For this review, take the finished solid that the model builds, in its own axes (mm). A direction names the side the tool comes from. Coordinates: 2 decimals unless noted, no trailing zeros. Order: outer loops, then holes, each group sorted by start corner. A loop starts at its lowest first (then second) coordinate and runs counter-clockwise, first axis right, second up. Notation, with made-up numbers: (-36.75, 34) -> (-16.75, 34) arc R28 cw to (-16.75, 72) -> close; hole circle Ø2 at (65.25, -10). An arc over 180 degrees is marked (long way). Write item = value, one per line. Start each with the question number.
1) Consider section A-A on x = -17.5. Give the boundary of the cut face in (y, z).
2) Consider section B-B on y = 22. Give the boundary of the cut face in (x, z).
3) Consider section C-C on x = 2. Give the boundary of the cut face in (y, z).
4) Draft analysis for pull direction X (two halves, no side actions). For faces 3 (the face through (57, 35.501, 15)), 4 (the face through (66.93, 42.4, -0.99)), 5 (the face through (-3.825, 36.621, 14.79)), state which applies: +X half, -X half, draft (parallel to the pull), parting line (faces both ways), or undercut.
5) Machinability: for faces 1 (the face through (66.9, -2.43, -0.99)), 2 (the face through (2, 40, 0)), which of the approach directions +Z, -Z, +X, -X, +Y, -Y give a long, thin tool a straight path to every point of the face, cutting with its end or side? Answer none if there is none.
6) Wall thickness on probe 1 along Y at (x, z) = (2, 2.6); probe 2 along X at (y, z) = (5.5, 19.5); probe 3 along Y at (x, z) = (43, 24): over which ranges is each line inside the solid? List them lowest first. Write a range as [from, to].
7) Insertion check: pin 1 Ø12 at (y, z) = (34.5, 8) entering from +X; pin 2 Ø9 at (y, z) = (25, 21.5) entering from +X; pin 3 Ø3 at (x, y) = (50.5, 39.5) entering from +Z; pin 4 Ø4 at (x, y) = (62.5, 22) entering from -Z. Each pin has a flat end and moves straight along its axis. Give the tip position at first contact, or say it passes through.
8) Consider section D-D on y = 33. Give the boundary of the cut face in (x, z).
from build123d import *

# Parameters (mm, degrees)
SKETCH_2_R          = 3.25
EXTRUDE_1_DEPTH     = 2
SKETCH_2_3_R        = 2
EXTRUDE_2_DEPTH     = 30
SKETCH_2_4_R        = 1.6
EXTRUDE_3_DEPTH     = 4
CUT_EXTRUDE_1_REACH = 80
SKETCH_3_R          = 2.5
SKETCH_3_R_2        = 2
CUT_EXTRUDE_2_REACH = 3.5


with BuildPart() as part:
    # Sketch 2 → Extrude 1 (new body)
    with BuildSketch(Plane.XY):
        with BuildLine():
            ThreePointArc((-20.5, 43.00095784), (-21.914213562, 42.415171403), (-22.5, 41.00095784))
            Line((-22.5, 41.00095784), (-22.5, -1))
            ThreePointArc((-22.5, -1), (-21.914213562, -2.414213562), (-20.5, -3))
            Line((-20.5, -3), (65.5, -3))
            ThreePointArc((65.5, -3), (66.914213562, -2.414213562), (67.5, -1))
            Line((67.5, -1), (67.5, 41.00095784))
            ThreePointArc((67.5, 41.00095784), (66.914213562, 42.415171403), (65.5, 43.00095784))
            Line((65.5, 43.00095784), (-20.5, 43.00095784))
        make_face()
        with Locations((-17.5, 22)):
            Circle(SKETCH_2_R, mode=Mode.SUBTRACT)
        with Locations((62.5, 22)):
            Circle(SKETCH_2_R, mode=Mode.SUBTRACT)
    extrude(amount=-EXTRUDE_1_DEPTH)

    # Sketch 2_3 → Extrude 2 (add)
    with BuildSketch(Plane.XY):
        with BuildLine():
            ThreePointArc((-10.601500464, -1), (-10.015714027, -2.414213562), (-8.601500464, -3))
            Line((-8.601500464, -3), (57.5, -3))
            ThreePointArc((57.5, -3), (61.5, 1), (57.5, 5))
            Line((57.5, 5), (55.5, 5))
            Line((55.5, 5), (55.5, 35.50095784))
            Line((55.5, 35.50095784), (58.590729836, 35.50095784))
            ThreePointArc((58.590729836, 35.50095784), (62.463713182, 38.50095784), (60.527221509, 43.00095784))
            Line((60.527221509, 43.00095784), (-8.601500464, 43.00095784))
            ThreePointArc((-8.601500464, 43.00095784), (-10.015714027, 42.415171403), (-10.601500464, 41.00095784))
            Line((-10.601500464, 41.00095784), (-10.601500464, -1))
        make_face()
        with Locations((-6.601500464, 1)):
            Circle(SKETCH_2_3_R, mode=Mode.SUBTRACT)
        with BuildLine():
            ThreePointArc((-3.137398849, -1), (-3.77307334, 3.828427125), (-8.601500464, 4.464101615))
            Line((-8.601500464, 4.464101615), (-8.601500464, 36.036856225))
            ThreePointArc((-8.601500464, 36.036856225), (-3.77307334, 36.672530716), (-3.137398849, 41.50095784))
            Line((-3.137398849, 41.50095784), (53.5, 41.50095784))
            Line((53.5, 41.50095784), (53.5, -1))
            Line((53.5, -1), (-3.137398849, -1))
        make_face(mode=Mode.SUBTRACT)
        with Locations((-6.601500464, 39.50095784)):
            Circle(SKETCH_2_3_R, mode=Mode.SUBTRACT)
        with Locations((57.5, 1)):
            Circle(SKETCH_2_3_R, mode=Mode.SUBTRACT)
        with Locations((58.590729836, 39.50095784)):
            Circle(SKETCH_2_3_R, mode=Mode.SUBTRACT)
    extrude(amount=EXTRUDE_2_DEPTH)

    # Sketch 2_4 → Extrude 3 (add)
    with BuildSketch(Plane.XY):
        with BuildLine():
            Line((4.872781496, 41.50095784), (-0.872781496, 41.50095784))
            ThreePointArc((-0.872781496, 41.50095784), (2, 35.99904216), (4.872781496, 41.50095784))
        make_face()
        with Locations((2, 39.5)):
            Circle(SKETCH_2_4_R, mode=Mode.SUBTRACT)
        with BuildLine():
            ThreePointArc((4.645751311, -1), (2, 6), (-0.645751311, -1))
            Line((-0.645751311, -1), (4.645751311, -1))
        make_face()
        with Locations((2, 2)):
            Circle(SKETCH_2_4_R, mode=Mode.SUBTRACT)
        with BuildLine():
            ThreePointArc((47.627218504, 41.50095784), (48.596140902, 36.56196897), (53.5, 37.695365466))
            Line((53.5, 37.695365466), (53.5, 41.50095784))
            Line((53.5, 41.50095784), (47.627218504, 41.50095784))
        make_face()
        with Locations((50.5, 39.5)):
            Circle(SKETCH_2_4_R, mode=Mode.SUBTRACT)
        with BuildLine():
            ThreePointArc((53.5, 4.645751311), (47.671572875, 4.828427125), (47.854248689, -1))
            Line((47.854248689, -1), (53.5, -1))
            Line((53.5, -1), (53.5, 4.645751311))
        make_face()
        with Locations((50.5, 2)):
            Circle(SKETCH_2_4_R, mode=Mode.SUBTRACT)
    extrude(amount=EXTRUDE_3_DEPTH)

    # Sketch 3 → Cut-Extrude 1 (cut, up to next)
    with BuildSketch(Plane(origin=(55.5, 0, 0), x_dir=(0, 0, -1), z_dir=(1, 0, 0)), mode=Mode.PRIVATE) as cut_extrude_1_sk1:
        with Locations((-30, 12.50095784)):
            Circle(SKETCH_3_R)
    cut_extrude_1_tool1 = extrude(cut_extrude_1_sk1.sketch, amount=-CUT_EXTRUDE_1_REACH, mode=Mode.PRIVATE) & part.part
    add(cut_extrude_1_tool1.solids().sort_by_distance((55.5, 12.500958, 30))[0], mode=Mode.SUBTRACT)
    # Sketch 3 → Cut-Extrude 1 (cut, up to next)
    with BuildSketch(Plane(origin=(55.5, 0, 0), x_dir=(0, 0, -1), z_dir=(1, 0, 0)), mode=Mode.PRIVATE) as cut_extrude_1_sk2:
        with Locations((-30, 28.50095784)):
            Circle(SKETCH_3_R_2)
    cut_extrude_1_tool2 = extrude(cut_extrude_1_sk2.sketch, amount=-CUT_EXTRUDE_1_REACH, mode=Mode.PRIVATE) & part.part
    add(cut_extrude_1_tool2.solids().sort_by_distance((55.5, 28.500958, 30))[0], mode=Mode.SUBTRACT)

    # Sketch 5 → Cut-Extrude 2 (cut, up to next)
    with BuildSketch(Plane.XZ.offset(-41.50095784), mode=Mode.PRIVATE) as cut_extrude_2_sk1:
        with BuildLine():
            Line((39.27567, 8.8), (47.49867, 8.8))
            Line((47.49867, 8.8), (47.49867, 6.3))
            ThreePointArc((47.49867, 6.3), (47.205776781, 5.592893219), (46.49867, 5.3))
            Line((46.49867, 5.3), (40.27567, 5.3))
            ThreePointArc((40.27567, 5.3), (39.568563219, 5.592893219), (39.27567, 6.3))
            Line((39.27567, 6.3), (39.27567, 8.8))
        make_face()
    cut_extrude_2_tool1 = extrude(cut_extrude_2_sk1.sketch, amount=-CUT_EXTRUDE_2_REACH, mode=Mode.PRIVATE) & part.part
    add(cut_extrude_2_tool1.solids().sort_by_distance((43.38717, 41.500958, 7.073111))[0], mode=Mode.SUBTRACT)


solid = part.part
Answer sheet:
q1.outline = (-3, -2) -> (18.75, -2) -> (18.75, 0) -> (-3, 0) -> close; (25.25, -2) -> (43, -2) -> (43, 0) -> (25.25, 0) -> close
q2.outline = (-22.5, -2) -> (-20.75, -2) -> (-20.75, 0) -> (-22.5, 0) -> close; (-14.25, -2) -> (59.25, -2) -> (59.25, 0) -> (55.5, 0) -> (55.5, 30) -> (53.5, 30) -> (53.5, 0) -> (-8.6, 0) -> (-8.6, 30) -> (-10.6, 30) -> (-10.6, 0) -> (-14.25, 0) -> close; (65.75, -2) -> (67.5, -2) -> (67.5, 0) -> (65.75, 0) -> close
q3.outline = (-3, -2) -> (43, -2) -> (43, 30) -> (41.5, 30) -> (41.5, 4) -> (41.1, 4) -> (41.1, 0) -> (37.9, 0) -> (37.9, 4) -> (36, 4) -> (36, 0) -> (6, 0) -> (6, 4) -> (3.6, 4) -> (3.6, 0) -> (0.4, 0) -> (0.4, 4) -> (-1, 4) -> (-1, 30) -> (-3, 30) -> close
q4.face_3 = draft
q4.face_4 = +X half
q4.face_5 = undercut
q5.face_1 = +Z, -Z, +X, -Y
q5.face_2 = +Z
q6.probe_1 = [-3, 0.4], [3.6, 6], [36, 37.9], [41.1, 43]
q6.probe_2 = [-10.6, -8.6], [53.5, 55.5]
q6.probe_3 = [-3, -1], [41.5, 43]
q7.pin_1 = 62.59
q7.pin_2 = 55.5
q7.pin_3 = 0
q7.pin_4 = through
q8.outline = (-22.5, -2) -> (67.5, -2) -> (67.5, 0) -> (55.5, 0) -> (55.5, 30) -> (53.5, 30) -> (53.5, 0) -> (-8.6, 0) -> (-8.6, 30) -> (-10.6, 30) -> (-10.6, 0) -> (-22.5, 0) -> close
